Source: CAD feature listing. Evaluate the final solid. Frame: model axes, mm. Face numbers are marked on the shaded views. A direction names the side the tool comes from. Coordinates: 2 decimals unless noted, no trailing zeros. Write each loop counter-clockwise with the first axis right and the second up, starting at its lowest first coordinate (ties: lowest second). Pieces come first, ordered by that corner, then holes. Notation, with made-up numbers: M -35,67 L 9,67 A31 ccw 9,97 Z; hole C 54.5,-3 d5. An arc over 180 degrees is marked long. Answer as CSV lines item,"result". Start each with the question number.
1. Section A-A on x = 0. Return the cut outline in (y, z), plus the area to 3 significant figures.
2. Section D-D on z = -3. Return the cut outline in (x, y).
3. Contact query for flat-ended pins moving along their axis: pin 1 Ø0.5 at (x, y) = (-0.5, 21.5) entering from -Z; pin 2 Ø4 at (y, z) = (7.5, -2) entering from +X; pin 3 Ø4 at (x, y) = (0.5, 12.5) entering from -Z. Output: stop coordinate, or through.
4. Line query: probe 1 along Y at (x, z) = (2.5, 0); probe 2 along X at (y, z) = (18.25, -1.25); probe 3 along Z at (x, y) = (1.5, 8). Output: solid intervals per line, ascending. Write a range as [from, to].
5. Reachability of the marked faces 1, 2 and 3 from +Z, -Z, +X, -X, +Y, -Y: full face, straight path, thin tool, end or side. Return the list, or none.
6. Section C-C on y = 6.25. Return the cut outline in (x, z).
7. Section B-B on z = 0.5. Return the cut outline in (x, y), plus the area to 3 significant figures.
Autodesk Inventor part; units mm, degrees
ref_plane "YZ Plane" through (0, 0, 0) normal (1, 0, 0) x (0, 1, 0)
ref_plane "XZ Plane" through (0, 0, 0) normal (0, 1, 0) x (-1, 0, 0)
ref_plane "XY Plane" through (0, 0, 0) normal (0, 0, 1) x (1, 0, 0)
sketch "Sketch1" plane through (0, 0, 0) normal (0, 1, 0) x (-1, 0, 0)
  circle A0 centre (0, 0) radius 1.95
  dimension "d0" = 3.9
extrude "Extrusion1" add sketch "Sketch1" along normal blind 20
sketch "Sketch2" plane through (0, 20, 0) normal (0, 1, 0) x (1, 0, 0)
  circle A0 centre (0, 0) radius 3.5
  dimension "d3" = 7
extrude "Extrusion2" add sketch "Sketch2" along normal blind 2
thread "Thread1"
sketch "Sketch3" plane through (0, 22, 0) normal (0, 1, 0) x (1, 0, 0)
  line L0 (0.866, 1.5) -> (1.7321, 0)
  line L1 (1.7321, 0) -> (0.866, -1.5)
  line L2 (0.866, -1.5) -> (-0.866, -1.5)
  line L3 (-0.866, -1.5) -> (-1.7321, 0)
  line L4 (-1.7321, 0) -> (-0.866, 1.5)
  line L5 (-0.866, 1.5) -> (0.866, 1.5)
  point P0 (0, 0)
  point P1 (0, 0)
  dimension "d8" = 3
extrude "Extrusion3" cut sketch "Sketch3" against normal blind 1
equation "\"BendRadius\" = Thickness"
equation "\"BendReliefWidth\" = Thickness"
equation "\"BendReliefDepth\" = 0.5 * Thickness"
equation "\"CornerReliefSize\" = 4 * Thickness"
equation "\"MinimumRemnant\" = 2 * Thickness"
equation "\"TransitionRadius\" = BendRadius"
equation "\"JacobiRadiusSize\" = BendRadius"
equation "\"GapSize\" = Thickness"
properties part number "perno_simple"
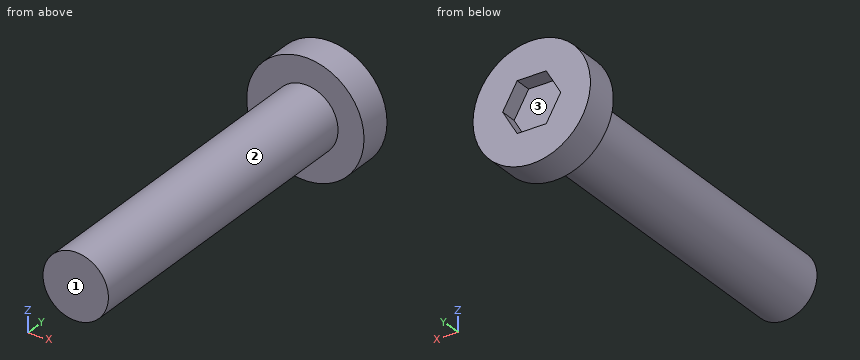
Values:
1,outline,"M 0,-1.95 L 20,-1.95 L 20,-3.5 L 22,-3.5 L 22,-1.5 L 21,-1.5 L 21,1.5 L 22,1.5 L 22,3.5 L 20,3.5 L 20,1.95 L 0,1.95 Z"
1,area,"89.0 mm²"
2,outline,"M -1.8,20 L 1.8,20 L 1.8,22 L -1.8,22 Z"
3,pin 1,"z = -3.49"
3,pin 2,"x = 1.95"
3,pin 3,"z = -1.95"
4,probe 1,"[20, 22]"
4,probe 2,"[-1.5, 1.5]"
4,probe 3,"[-1.25, 1.25]"
5,face 1,"+Z, -Z, +X, -X, -Y"
5,face 2,"-Y"
5,face 3,"+Y"
6,outline,"C 0,0 d3.9"
7,outline,"M -3.46,20 L -1.88,20 L -1.88,0 L 1.88,0 L 1.88,20 L 3.46,20 L 3.46,22 L 1.44,22 L 1.44,21 L -1.44,21 L -1.44,22 L -3.46,22 Z"
7,area,"86.4 mm²"
